Geometry: final body of the model. Coordinates: model frame, mm. A direction names the side the tool comes from. Give positions to 0.01 mm unless a question says otherwise; leave off trailing zeros. Order: outer loops, then holes, each group sorted by start corner. A loop starts at its lowest first (then second) coordinate and runs counter-clockwise, first axis right, second up. Notation, with made-up numbers: (-1.5, -22.75) - (20.5, -22.75) arc R30 ccw to (20.5, 7.25) - close; hole circle Ø11 at (32.5, -32.75). An arc over 180 degrees is marked (long way). One line per item, written item: value.
```python
from build123d import *

# Parameters (mm, degrees)
F0_W           = 25
F0_H           = 12
F1_DEPTH       = 1
F2_T1_DEPTH    = 56.4409720866
F1_FACE_W      = 25
F1_FACE_H      = 12
F3_DEPTH       = 1
F4_W           = 20
F4_H           = 9
F5_DEPTH       = 15
F6_W           = 5
F6_H           = 8
F7_DEPTH       = 4
F10_DEPTH      = 10
F10_DEPTH_BACK = 2
F11_R          = 0.5
F12_W          = 22.0358781517
F12_H          = 9.327288717
F12_W_2        = 5
F12_H_2        = 8
F12_W_3        = 7.4061334931
F13_DEPTH      = 3.5
F16_R          = 1
F18_DEPTH      = 4
F19_R          = 0.19999


# Not quite as in the source:
# - a fillet or chamfer that OpenCascade refuses, or shapes differently, is made with other operations: its cross-section is extruded or revolved along the edge and cut away or added
# - a fillet or chamfer is up to 0.001 mm smaller than in the source, because OpenCascade refuses the exact size
# - the program builds the solid bodies; features that only make, move or delete a surface that nothing else refers to are left out


with BuildPart() as f1:
    # F0 (on Top) → F1 (new body)
    with BuildSketch(Plane.XY):
        Rectangle(F0_W, F0_H)
    extrude(amount=F1_DEPTH)

    # F2: fillet of radius 40 on 2 edges, made by hand

    # F2_s2 → F2_t1 (cut)
    with BuildSketch(Plane.XZ.offset(-28.2204860433)):
        with BuildLine():
            add(Edge.make_bspline(
                [(12.5, 0), (8.1121571864, 1), (3.6118055827, 1)],
                knots=[0, 0, 0, 1, 1, 1], degree=2, weights=[1, 1, 1]))
            Line((3.6118055827, 1), (3.6118055827, 1.8))
            Line((3.6118055827, 1.8), (12.5, 1.8))
            Line((12.5, 1.8), (13.3, 1))
            ThreePointArc((13.3, 1), (13.3, 0.5), (12.6777638883, 0.78))
            Line((12.6777638883, 0.78), (12.5, 0))
        make_face()
        with BuildLine():
            add(Edge.make_bspline(
                [(-12.5, 0), (-8.1121571864, 1), (-3.6118055827, 1)],
                knots=[0, 0, 0, 1, 1, 1], degree=2, weights=[1, 1, 1]))
            Line((-3.6118055827, 1), (-3.6118055827, 1.8))
            Line((-3.6118055827, 1.8), (-12.5, 1.8))
            Line((-12.5, 1.8), (-13.3, 1))
            ThreePointArc((-13.3, 1), (-13.3, 0.5), (-12.6777638883, 0.78))
            Line((-12.6777638883, 0.78), (-12.5, 0))
        make_face()
    extrude(amount=F2_T1_DEPTH, mode=Mode.SUBTRACT)

    # F1_face (on face) + F0 (on Top) → F3 (join)
    with BuildSketch(Plane(origin=(0, 0, 0), x_dir=(1, 0, 0), z_dir=(0, 0, -1))):
        Rectangle(F1_FACE_W, F1_FACE_H)
    with BuildSketch(Plane.XY):
        Rectangle(F0_W, F0_H)
    extrude(amount=F3_DEPTH, dir=(0, 0, -1))

    # F4 (on face) → F5 (join)
    with BuildSketch(Plane(origin=(0, 0, -1), x_dir=(1, 0, 0), z_dir=(0, 0, -1))):
        Rectangle(F4_W, F4_H)
    extrude(amount=F5_DEPTH)

    # F6 (on face) → F7 (join)
    with BuildSketch(Plane.XY.offset(1)):
        Rectangle(F6_W, F6_H)
    extrude(amount=F7_DEPTH)

    # F9 (on face) → F10 (join, two sides)
    with BuildSketch(Plane.XZ.offset(4)) as f10_sk:
        Polygon((-12.8228797714, 4.2615274688), (0, 1.6069198027), (12.1771202286, 4.2615274688), (12.1771202286, 5.2615274688), (-12.8228797714, 5.2615274688), align=None)
        with BuildLine():
            Line((-12.8228797714, 5.2615274688), (12.1771202286, 5.2615274688))
            ThreePointArc((12.1771202286, 5.2615274688), (-0.3228797714, 6.9123152663), (-12.8228797714, 5.2615274688))
        make_face()
    extrude(amount=-F10_DEPTH)
    extrude(f10_sk.sketch, amount=F10_DEPTH_BACK)

    # F11
    f11_edges = [f1.edges().sort_by_distance(p)[0] for p in [
        (-0.32288, 6, 6.912315),
        (-12.82288, 0, 5.261527),
        (-0.32288, -6, 6.912315),
        (12.17712, 0, 5.261527),
        (12.17712, -6, 4.761527),
        (-12.82288, -6, 4.761527),
        (-12.82288, 6, 4.761527),
        (12.17712, 6, 4.761527),
    ]]
    fillet(f11_edges, radius=F11_R)

    # F12 (on face) → F13 (cut)
    with BuildSketch(Plane.XY.offset(1)):
        Rectangle(F12_W, F12_H)
        Rectangle(F12_W_2, F12_H_2, mode=Mode.SUBTRACT)
        with Locations((-7.3148723293, 0)):
            Rectangle(F12_W_3, F12_H)
    extrude(amount=F13_DEPTH, mode=Mode.SUBTRACT)

    # F16
    f16_edges = [f1.edges().sort_by_distance(p)[0] for p in [
        (-10, -4.5, -8.5),
        (10, -4.5, -8.5),
        (-10, 4.5, -8.5),
        (10, 4.5, -8.5),
    ]]
    fillet(f16_edges, radius=F16_R)

    # F17 (on Front) → F18 (cut, symmetric)
    with BuildSketch(Plane.XZ):
        with BuildLine():
            Line((-13, 7.209603209), (-13, 5.0062067558))
            ThreePointArc((-13, 5.0062067558), (0.0125633764, 6.7111419558), (13, 4.8243193332))
            Line((13, 4.8243193332), (13, 7.209603209))
            Line((13, 7.209603209), (-13, 7.209603209))
        make_face()
    extrude(amount=F18_DEPTH, both=True, mode=Mode.SUBTRACT)

    # F19 (radius 0.2 in the source; OpenCascade refuses exactly that, so slightly less here)
    f19_edges = [f1.edges().sort_by_distance(p)[0] for p in [
        (-0.32288, -4, 6.912315),
        (-0.32288, 4, 6.912315),
    ]]
    fillet(f19_edges, radius=F19_R)


solid = f1.part
```
1) Section A-A, the plane z = 2.5. Return loops of the section in (x, y).
Answers below:
outline: (-4.31, -6) - (4.1, -6) - (4.1, -4.66) - (-4.31, -4.66) - close; (-4.31, 4.66) - (4.1, 4.66) - (4.1, 6) - (-4.31, 6) - close; (-2.5, -4) - (2.5, -4) - (2.5, 4) - (-2.5, 4) - close
2) Material intervals for line 1 along Y through (x, z) = (-1, 3.5); line 2 along Y through (x, z) = (-7.5, 3.25); line 3 along X through (y, z) = (2.75, 4.75), sorted ascending.
Answers below:
line 1: -6 to -4.66, -4 to 4, 4.66 to 6
line 2: -6 to -4.66, 4.66 to 6
line 3: -12.82 to 12.18
3) Section B-B, the plane z = -1.5. Return loops of the section in (x, y), then the cut area to 3 significant figures.
Answers below:
outline: (-10, -3.5) arc R1 ccw to (-9, -4.5) - (9, -4.5) arc R1 ccw to (10, -3.5) - (10, 3.5) arc R1 ccw to (9, 4.5) - (-9, 4.5) arc R1 ccw to (-10, 3.5) - close
area: 179 mm^2
4) Mould query, pull axis X, two halves, no side actions, for faces 4 (the face through (0, 0, -16)), 5 (the face through (-9.715, -4.199, -8.605)), 6 (the face through (0, 4.664, 3)). Classes: released by +X, released by -X, zero draft, split by the parting line, or undercut.
Answers below:
face 4: zero draft
face 5: released by -X
face 6: undercut
5) First-contact query: pin 1 (1.5 mm diameter, centred on y = 3, z = -13, fed in from -X); pin 2 (1.5 mm diameter, centred on x = -2, z = -7, fed in from +Y); pin 3 (4.5 mm diameter, centred on x = -3, z = -5.5, fed in from -Y). Flat tips, straight axial feed; report the tip coordinate or a pass-through.
Answers below:
pin 1: x = -10
pin 2: y = 4.5
pin 3: y = -4.5
6) Set-up query: faces 1 (the face through (-2.5, 0, 3)), 2 (the face through (10, 0, -8)), 3 (the face through (0, 5, -1)). Return all of +Z, -Z, +X, -X, +Y, -Y with unobstructed straight access to the full face (end or side cutting, diameter ignored); none if empty.
Answers below:
face 1: none
face 2: -Z, +X, +Y, -Y
face 3: -Z
